Autodesk Inventor part; units mm, degrees
ref_plane "YZ Plane" through (0, 0, 0) normal (1, 0, 0) x (0, 1, 0)
ref_plane "XZ Plane" through (0, 0, 0) normal (0, 1, 0) x (-1, 0, 0)
ref_plane "XY Plane" through (0, 0, 0) normal (0, 0, 1) x (1, 0, 0)
sketch "Sketch1" plane through (0, 0, 0) normal (0, 1, 0) x (-1, 0, 0)
  arc A0 (-4.5172, 1.6395) -> (-5.4471, 3.8845) centre (-7.6922, 1.6395) ccw
  line L0 (-8.7553, 7.1927) -> (-5.4471, 3.8845)
  arc A1 (-8.7553, 7.1927) -> (-10.4897, 6.4823) centre (-9.4737, 6.4743) ccw
  arc A2 (-10.4897, 6.4823) -> (6.4823, -10.4897) centre (6.35, 6.35) ccw
  arc A3 (6.4823, -10.4897) -> (7.1927, -8.7553) centre (6.4743, -9.4737) ccw
  line L1 (3.8845, -5.4471) -> (7.1927, -8.7553)
  arc A4 (3.8845, -5.4471) -> (1.6395, -4.5172) centre (1.6395, -7.6922) ccw
  line L2 (-2.3074, -4.5172) -> (1.6395, -4.5172)
  arc A5 (-4.5172, -2.3074) -> (-2.3074, -4.5172) centre (-2.3074, -2.3074) ccw
  line L3 (-4.5172, 1.6395) -> (-4.5172, -2.3074)
  arc A6 (-2.2319, 1.3405) -> (-2.2319, -1.3405) centre (0, 0) ccw
  line L4 (-2.8605, -1.9692) -> (-2.2319, -1.3405)
  arc A7 (-2.8605, -1.9692) -> (-1.9692, -2.8605) centre (-2.4696, -2.4696) ccw
  line L5 (-1.3405, -2.2319) -> (-1.9692, -2.8605)
  arc A8 (-1.3405, -2.2319) -> (1.3405, -2.2319) centre (0, 0) ccw
  line L6 (1.9692, -2.8605) -> (1.3405, -2.2319)
  arc A9 (1.9692, -2.8605) -> (2.8605, -1.9692) centre (2.4696, -2.4696) ccw
  line L7 (2.2319, -1.3405) -> (2.8605, -1.9692)
  arc A10 (2.2319, -1.3405) -> (2.2319, 1.3405) centre (0, 0) ccw
  line L8 (2.8605, 1.9692) -> (2.2319, 1.3405)
  arc A11 (2.8605, 1.9692) -> (1.9692, 2.8605) centre (2.4696, 2.4696) ccw
  line L9 (1.3405, 2.2319) -> (1.9692, 2.8605)
  arc A12 (1.3405, 2.2319) -> (-1.3405, 2.2319) centre (0, 0) ccw
  line L10 (-1.9692, 2.8605) -> (-1.3405, 2.2319)
  arc A13 (-1.9692, 2.8605) -> (-2.8605, 1.9692) centre (-2.4696, 2.4696) ccw
  line L11 (-2.2319, 1.3405) -> (-2.8605, 1.9692)
  arc A14 (12.7, -4.3561) -> (10.4902, -4.3561) centre (11.5951, -4.3561) ccw
  line L12 (12.7, -4.3561) -> (12.7, -10.5918)
  arc A15 (10.5918, -12.7) -> (12.7, -10.5918) centre (10.5918, -10.5918) ccw
  line L13 (10.5918, -12.7) -> (6.35, -12.7)
  arc A16 (-12.7, 6.35) -> (6.35, -12.7) centre (6.35, 6.35) ccw
  line L14 (-12.7, 6.35) -> (-12.7, 10.5918)
  arc A17 (-10.5918, 12.7) -> (-12.7, 10.5918) centre (-10.5918, 10.5918) ccw
  line L15 (-10.5918, 12.7) -> (-4.3561, 12.7)
  arc A18 (-4.3561, 10.4902) -> (-4.3561, 12.7) centre (-4.3561, 11.5951) ccw
  line L16 (-4.3561, 10.4902) -> (-6.4749, 10.4902)
  arc A19 (-6.4749, 10.4902) -> (-7.1933, 8.7558) centre (-6.4749, 9.4742) ccw
  line L17 (-7.1933, 8.7558) -> (-3.8846, 5.4471)
  arc A20 (-3.8846, 5.4471) -> (-1.6396, 4.5172) centre (-1.6396, 7.6922) ccw
  line L18 (-1.6396, 4.5172) -> (1.6396, 4.5172)
  arc A21 (1.6396, 4.5172) -> (3.8846, 5.4471) centre (1.6396, 7.6922) ccw
  line L19 (3.8846, 5.4471) -> (7.1933, 8.7558)
  arc A22 (7.1933, 8.7558) -> (6.4749, 10.4902) centre (6.4749, 9.4742) ccw
  line L20 (6.4749, 10.4902) -> (4.3561, 10.4902)
  arc A23 (4.3561, 12.7) -> (4.3561, 10.4902) centre (4.3561, 11.5951) ccw
  line L21 (4.3561, 12.7) -> (10.5918, 12.7)
  arc A24 (12.7, 10.5918) -> (10.5918, 12.7) centre (10.5918, 10.5918) ccw
  line L22 (12.7, 10.5918) -> (12.7, 4.3561)
  arc A25 (10.4902, 4.3561) -> (12.7, 4.3561) centre (11.5951, 4.3561) ccw
  line L23 (10.4902, 4.3561) -> (10.4902, 6.4749)
  arc A26 (10.4902, 6.4749) -> (8.7558, 7.1933) centre (9.4742, 6.4749) ccw
  line L24 (8.7558, 7.1933) -> (5.4471, 3.8846)
  arc A27 (5.4471, 3.8846) -> (4.5172, 1.6396) centre (7.6922, 1.6396) ccw
  line L25 (4.5172, 1.6396) -> (4.5172, -1.6396)
  arc A28 (4.5172, -1.6396) -> (5.4471, -3.8846) centre (7.6922, -1.6396) ccw
  line L26 (5.4471, -3.8846) -> (8.7558, -7.1933)
  arc A29 (8.7558, -7.1933) -> (10.4902, -6.4749) centre (9.4742, -6.4749) ccw
  line L27 (10.4902, -6.4749) -> (10.4902, -4.3561)
  point P0 (0, 0)
  dimension "d0" = 1.1049
  dimension "d1" = 2.1082
  dimension "d2" = 1.016
  dimension "d3" = 3.175
  dimension "d4" = 19.05
  dimension "d5" = 16.8402
  dimension "d6" = 0.635
  dimension "d7" = 2.6035
  dimension "d8" = 2.6035
  dimension "d9" = 2.6035
  dimension "d10" = 2.6035
  dimension "d11" = 2.2098
  dimension "d12" = 45
  dimension "d13" = 45
  dimension "d14" = 45
  dimension "d15" = 45
  dimension "d16" = 45
  dimension "d17" = 45
  dimension "d18" = 90
  dimension "d19" = 45
  dimension "d20" = 90
  dimension "d21" = 90
  dimension "d22" = 90
  dimension "d23" = 8.1828
  dimension "d24" = 17.2172
  dimension "d25" = 25.4
  dimension "d26" = 25.4
  dimension "d27" = 17.2172
  dimension "d28" = 8.1828
  dimension "d29" = 2.2096
  dimension "d30" = 1.7351
  dimension "d31" = 0.4746
  dimension "d32" = 1.7352
  dimension "d33" = 0.4746
  dimension "d34" = 2.2097
  dimension "d35" = 12.7
  dimension "d36" = 12.7
  dimension "d37" = 10.4902
  dimension "d38" = 12.7
  dimension "d39" = 1.1048
  dimension "d40" = 1.1048
  dimension "d41" = 1.1049
  dimension "d42" = 0.6303
  dimension "d43" = 0.6303
  dimension "d44" = 0.6303
  dimension "d45" = 0.6303
  dimension "d46" = 10.4902
  dimension "d47" = 1.1049
  dimension "d48" = 12.7
  dimension "d49" = 17.0561
  dimension "d50" = 8.3439
  dimension "d51" = 8.3439
  dimension "d52" = 9.8395
  dimension "d53" = 9.8395
  dimension "d54" = 10.2304
  dimension "d55" = 10.2304
  dimension "d56" = 10.4681
  dimension "d57" = 10.4681
  dimension "d58" = 14.6692
  dimension "d59" = 14.6692
  dimension "d60" = 15.1696
  dimension "d61" = 15.1696
  dimension "d62" = 17.0561
extrude "Extrusion1" add sketch "Sketch1" along normal mid plane 25.4
properties part number "1012-S-BLACK-FB" material "6105-T5"
Can you work these out from the model? Positions are in its coordinate system, mm. A direction names the side the tool comes from. Coordinates: 2 decimals unless noted, no trailing zeros. Write each loop counter-clockwise with the first axis right and the second up, starting at its lowest first coordinate (ties: lowest second). Pieces come first, ordered by that corner, then holes. Notation, with made-up numbers: (84, -32.75) -> (135, -32.75) arc R20 cw to (135, -2.75) -> close; hole circle Ø4 at (-13, -18.75). An arc over 180 degrees is marked (long way). Write item = value, one per line.
(1) Imagine slicing it at A-A (z = -10). Please give me the cut outline in (x, y), and give its area (3 significant figures).
Verdict:
outline = (-12.7, -12.7) -> (-7.34, -12.7) -> (-7.34, 12.7) -> (-12.7, 12.7) -> close; (-2.32, -12.7) -> (3.43, -12.7) -> (3.43, 12.7) -> (-2.32, 12.7) -> close
area = 282 mm^2
(2) If I drill on probe 1 along X at (y, z) = (1.75, -5); probe 2 along X at (y, z) = (4.25, -2.75); probe 3 along Z at (x, y) = (-6, 8), over which ranges is the centre line in solid material (lowest first)?
Verdict:
probe_1 = -12.7 to -10.49, -6.56 to -3.32, 6.09 to 8.95
probe_2 = -4.72 to -3.04, -1.86 to 1.86, 3.04 to 4.47, 7.82 to 10.39
probe_3 = -12.7 to -10.49, -7.56 to -4.44, 4.44 to 7.56, 10.49 to 12.7
(3) Thinking about a two-plate mould opening in Z: for faces 1 (the face through (-7, 0, 12.7)), 2 (the face through (-2.603, -0.178, 0.02)), 3 (the face through (-12.7, 0, 8)), which applies, +Z half, -Z half, draft (parallel to the pull), parting line (faces both ways), or undercut?
Verdict:
face_1 = +Z half
face_2 = undercut
face_3 = draft
(4) Imagine slicing it at D-D (x = 11.25). Please give me the cut outline in (y, z), and give its area (3 significant figures).
Verdict:
outline = (-12.7, -0.94) -> (12.7, -0.94) -> (12.7, 12.59) -> (-12.7, 12.59) -> close
area = 344 mm^2
(5) On a 3-axis mill with a long thin cutter (end or side, diameter ignored), from which of +Z, -Z, +X, -X, +Y, -Y can I reach the whole of each face in a straight line? I mean faces 4 (the face through (-11.57, -0.18, -3.25)), 5 (the face through (0, 12.7, 3)). Say none if no direction works.
Verdict:
face_4 = +Y, -Y
face_5 = +Z, -Z, +X, -X, +Y
(6) Imagine slicing it at B-B (x = -8.25). Please give me the cut outline in (y, z).
Verdict:
outline = (-12.7, -12.7) -> (12.7, -12.7) -> (12.7, -6.69) -> (-12.7, -6.69) -> close; (-12.7, 6.69) -> (12.7, 6.69) -> (12.7, 12.7) -> (-12.7, 12.7) -> close
(7) For pin 1 (1.2 mm diameter, centred on x = -0.5, y = -1, fed in from -Z); pin 2 (1.2 mm diameter, centred on y = -5.5, z = 0.5, fed in from +X); pin 3 (5 mm diameter, centred on x = 4.5, y = 9.5, fed in from -Z), each with a flat end and sliding along its axis, tell me the tip position at first contact or that it passes through.
Verdict:
pin_1 = -11.96
pin_2 = 11.96
pin_3 = -10.77
(8) Imagine slicing it at C-C (y = 5). State how many separate pieces and enclosed holes the cut face has, and give its area (3 significant figures).
Verdict:
separate_pieces = 1
enclosed_holes = 2
area = 271 mm^2
